Geometry: final body of the model. Coordinates: model frame, mm. Face numbers are marked on the shaded views. Round coordinates to 2 decimals unless told otherwise and drop trailing zeros. Loops run counter-clockwise (first coordinate to the right, second up) from the corner with the lowest first, then second, coordinate; pieces in that order, holes last. Notation, with made-up numbers: (-39.5, 9) -> (9.5, 9) arc R19 cw to (9.5, 24) -> close; hole circle Ø9 at (22.25, 67). An arc over 180 degrees is marked (long way). Answer in a Markdown table with one row per item.
```python
from build123d import *

# Parameters (mm, degrees)
F0_R     = 6.35
F1_DEPTH = 12.7


with BuildPart() as f1:
    # F0 (on Right) → F1 (new body)
    with BuildSketch(Plane.YZ):
        with BuildLine():
            Line((37.457174, 25.4), (-25.4, 25.4))
            Line((-25.4, 25.4), (-25.4, 0))
            ThreePointArc((-25.4, 0), (-4.784957, -24.945224), (23.59718, -9.398569))
            Line((23.59718, -9.398569), (37.457174, 25.4))
        make_face()
        Circle(F0_R, mode=Mode.SUBTRACT)
    extrude(amount=F1_DEPTH)


solid = f1.part
```
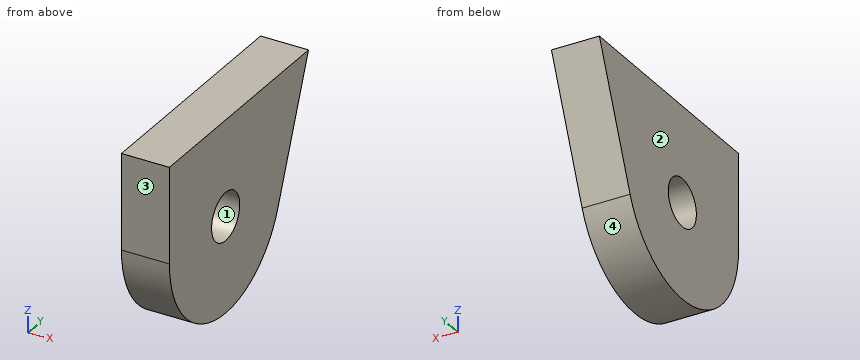
Item 1: Cut plane A-A (y = 0). Output: boundary loops of the cut face in (x, z).
Answer:
| item | result |
|---|---|
| outline | (0, -25.4) -> (12.7, -25.4) -> (12.7, -6.35) -> (0, -6.35) -> close; (0, 6.35) -> (12.7, 6.35) -> (12.7, 25.4) -> (0, 25.4) -> close |
Item 2: Pin query (flat end, axial travel): pin 1 Ø1 at (x, z) = (5, -11) entering from +Y; pin 2 Ø3 at (x, z) = (3, 2) entering from +Y; pin 3 Ø3 at (x, y) = (5, 17) entering from -Z. Return the tip coordinate at first contact, or that it passes through.
Answer:
| item | result |
|---|---|
| pin 1 | stops at y = 23.13 |
| pin 2 | stops at y = 28.73 |
| pin 3 | stops at z = -20.12 |
Item 3: Draft query along Y for the marked faces 1, 2, 3 and 4. Return one class per face: pulls with the +Y half, pulls with the -Y half, needs draft (parallel to the pull), parting line crosses it, or undercut.
Answer:
| item | result |
|---|---|
| face 1 | undercut |
| face 2 | needs draft |
| face 3 | pulls with the -Y half |
| face 4 | parting line crosses it |
Item 4: Cut plane B-B (x = 7). Output: boundary loops of the cut face in (y, z), then the cut area to 3 significant figures.
Answer:
| item | result |
|---|---|
| outline | (-25.4, 0) arc R25.4 ccw to (23.6, -9.4) -> (37.46, 25.4) -> (-25.4, 25.4) -> close; hole circle Ø12.7 at (0, 0) |
| area | 2,360 mm² |
Item 5: Cut plane C-C (y = -15.5). Output: boundary loops of the cut face in (x, z).
Answer:
| item | result |
|---|---|
| outline | (0, -20.12) -> (12.7, -20.12) -> (12.7, 25.4) -> (0, 25.4) -> close |
Item 6: Line query: probe 1 along Z at (x, y) = (5.75, 0); probe 2 along Y at (x, z) = (9, -18.5); probe 3 along Y at (x, z) = (11, 1). Output: solid intervals per line, ascending. Write a range as [from, to].
Answer:
| item | result |
|---|---|
| probe 1 | z = [-25.4, -6.35], [6.35, 25.4] |
| probe 2 | y = [-17.4, 17.4] |
| probe 3 | y = [-25.4, -6.27], [6.27, 27.74] |
Item 7: Cut plane D-D (z = -19). Output: boundary loops of the cut face in (x, y), then the cut area to 3 significant figures.
Answer:
| item | result |
|---|---|
| outline | (0, -16.86) -> (12.7, -16.86) -> (12.7, 16.86) -> (0, 16.86) -> close |
| area | 428 mm² |
